Source: CAD feature listing. Evaluate the final solid. Frame: model axes, mm. A direction names the side the tool comes from. Coordinates: 2 decimals unless noted, no trailing zeros. Order: outer loops, then holes, each group sorted by start corner. A loop starts at its lowest first (then second) coordinate and runs counter-clockwise, first axis right, second up. Notation, with made-up numbers: (57, 47) -> (102, 47) arc R33 ccw to (102, 76) -> close; hole circle Ø6 at (-10, 80.5). An arc over 180 degrees is marked (long way). Put each result on its own line as item: value.
from build123d import *

# Parameters (mm, degrees)
SKETCH1_W                 = 465.838
SKETCH1_H                 = 365.232
BOSS_EXTRUDE1_DEPTH       = 3.175
SKETCH2_W                 = 465.838
SKETCH2_H                 = 365.232
SKETCH2_W_2               = 459.488
SKETCH2_H_2               = 47.625
SKETCH2_W_3               = 89.789
SKETCH2_H_3               = 308.082
SKETCH2_W_4               = 87.632
BOSS_EXTRUDE2_DEPTH       = 200.6
BOSS_EXTRUDE5_OUTLINE_W   = 87.632
BOSS_EXTRUDE5_OUTLINE_H   = 308.082
BOSS_EXTRUDE5_OUTLINE_W_2 = 89.789
BOSS_EXTRUDE5_DEPTH       = 38.1
CUT_EXTRUDE2_DEPTH        = 35
BOSS_EXTRUDE6_DEPTH       = 30.8
CUT_EXTRUDE3_DEPTH        = 579.469838561
SKETCH10_W                = 34.036
SKETCH10_H                = 101.6
SKETCH10_W_2              = 50.8
SKETCH10_H_2              = 34.036
BOSS_EXTRUDE7_DEPTH       = 3.175


# Read off the part's stored shape, not the designer's step: Boss-Extrude5
with BuildPart() as part:
    # Sketch1 → Boss-Extrude1 (new body)
    with BuildSketch(Plane.XY):
        with Locations((-46.4825, -25.4)):
            Rectangle(SKETCH1_W, SKETCH1_H)
    extrude(amount=BOSS_EXTRUDE1_DEPTH)

    # Sketch2 → Boss-Extrude2 (add)
    with BuildSketch(Plane.XY.offset(3.175)):
        with Locations((-46.4825, -25.4)):
            Rectangle(SKETCH2_W, SKETCH2_H)
        with Locations((-46.4825, -181.0285)):
            Rectangle(SKETCH2_W_2, SKETCH2_H_2, mode=Mode.SUBTRACT)
        with Locations((138.367, 0)):
            Rectangle(SKETCH2_W_3, SKETCH2_H_3, mode=Mode.SUBTRACT)
        with Locations((45.403, 0)):
            Rectangle(SKETCH2_W_3, SKETCH2_H_3, mode=Mode.SUBTRACT)
        with Locations((-47.561, 0)):
            Rectangle(SKETCH2_W_3, SKETCH2_H_3, mode=Mode.SUBTRACT)
        with Locations((-140.525, 0)):
            Rectangle(SKETCH2_W_3, SKETCH2_H_3, mode=Mode.SUBTRACT)
        with Locations((-232.4105, 0)):
            Rectangle(SKETCH2_W_4, SKETCH2_H_3, mode=Mode.SUBTRACT)
    extrude(amount=BOSS_EXTRUDE2_DEPTH)

    # Boss-Extrude5 outline → Boss-Extrude5 (add)
    with BuildSketch(Plane.XY.offset(203.775)):
        Polygon((183.2615, -208.016), (186.4365, -208.016), (186.4365, 157.216), (-279.4015, 157.216), (-279.4015, -208.016), (-276.2265, -208.016), (-276.2265, -157.216), (183.2615, -157.216), align=None)
        with Locations((-232.4105, 0)):
            Rectangle(BOSS_EXTRUDE5_OUTLINE_W, BOSS_EXTRUDE5_OUTLINE_H, mode=Mode.SUBTRACT)
        with Locations((-140.525, 0)):
            Rectangle(BOSS_EXTRUDE5_OUTLINE_W_2, BOSS_EXTRUDE5_OUTLINE_H, mode=Mode.SUBTRACT)
        with Locations((-47.561, 0)):
            Rectangle(BOSS_EXTRUDE5_OUTLINE_W_2, BOSS_EXTRUDE5_OUTLINE_H, mode=Mode.SUBTRACT)
        with Locations((45.403, 0)):
            Rectangle(BOSS_EXTRUDE5_OUTLINE_W_2, BOSS_EXTRUDE5_OUTLINE_H, mode=Mode.SUBTRACT)
        with Locations((138.367, 0)):
            Rectangle(BOSS_EXTRUDE5_OUTLINE_W_2, BOSS_EXTRUDE5_OUTLINE_H, mode=Mode.SUBTRACT)
    extrude(amount=BOSS_EXTRUDE5_DEPTH)

    # Sketch7 → Cut-Extrude2 (cut)
    with BuildSketch(Plane.XY.offset(241.875)):
        Polygon((-185.4195, -154.041), (-185.4195, 154.041), (-188.5945, 154.041), (-188.5945, -154.041), (-276.2265, -154.041), (-276.2265, -157.216), (183.2615, -157.216), (183.2615, -154.041), (93.4725, -154.041), (93.4725, 154.041), (90.2975, 154.041), (90.2975, -154.041), (0.5085, -154.041), (0.5085, 154.041), (-2.6665, 154.041), (-2.6665, -154.041), (-92.4555, -154.041), (-92.4555, 154.041), (-95.6305, 154.041), (-95.6305, -154.041), align=None)
    extrude(amount=-CUT_EXTRUDE2_DEPTH, mode=Mode.SUBTRACT)

    # Sketch8 → Boss-Extrude6 (add)
    with BuildSketch(Plane.XY.offset(241.875)):
        Polygon((183.2615, 154.041), (183.2615, -208.016), (186.4365, -208.016), (186.4365, 157.216), (-279.4015, 157.216), (-279.4015, -208.016), (-276.2265, -208.016), (-276.2265, 154.041), align=None)
    extrude(amount=BOSS_EXTRUDE6_DEPTH)

    # Sketch9 → Cut-Extrude3 (cut, through all)
    with BuildSketch(Plane(origin=(186.4365, 0, 0), x_dir=(0, 0, -1), z_dir=(1, 0, 0))):
        Polygon((-272.675, -208.016), (-215.525, -208.016), (-272.675, -131.816), align=None)
        Polygon((-272.675, 157.216), (-272.675, 81.016), (-215.525, 157.216), align=None)
    extrude(amount=-CUT_EXTRUDE3_DEPTH, mode=Mode.SUBTRACT)

    # Sketch10 → Boss-Extrude7 (add)
    with BuildSketch(Plane.XY):
        with Locations((203.4545, 106.416)):
            Rectangle(SKETCH10_W, SKETCH10_H)
        with Locations((203.4545, -106.416)):
            Rectangle(SKETCH10_W, SKETCH10_H)
        with Locations((161.0365, 174.234)):
            Rectangle(SKETCH10_W_2, SKETCH10_H_2)
    boss_extrude7 = extrude(amount=BOSS_EXTRUDE7_DEPTH)

    # Mirror1: Boss-Extrude7 across plane
    add(boss_extrude7.mirror(Plane.ZY.offset(46.4825)))


solid = part.part
1. Cut plane D-D on y = -79. Output: boundary loops of the cut face in (x, z) (1 decimal).
Numbers:
outline: (-313.4, 0) -> (220.5, 0) -> (220.5, 3.2) -> (186.4, 3.2) -> (186.4, 272.7) -> (183.3, 272.7) -> (183.3, 3.2) -> (93.5, 3.2) -> (93.5, 206.9) -> (90.3, 206.9) -> (90.3, 3.2) -> (0.5, 3.2) -> (0.5, 206.9) -> (-2.7, 206.9) -> (-2.7, 3.2) -> (-92.5, 3.2) -> (-92.5, 206.9) -> (-95.6, 206.9) -> (-95.6, 3.2) -> (-185.4, 3.2) -> (-185.4, 206.9) -> (-188.6, 206.9) -> (-188.6, 3.2) -> (-276.2, 3.2) -> (-276.2, 272.7) -> (-279.4, 272.7) -> (-279.4, 3.2) -> (-313.4, 3.2) -> close
2. Cut plane C-C on z = 246.5. Output: boundary loops of the cut face in (x, y), plus the area to 3 significant figures.
Numbers:
outline: (-279.4, -166.72) -> (-276.23, -166.72) -> (-276.23, 115.92) -> (-279.4, 115.92) -> close; (183.26, -166.72) -> (186.44, -166.72) -> (186.44, 115.92) -> (183.26, 115.92) -> close
area: 1,790 mm2
3. Set-up query: faces 1 (the flat face through (90.298, -2, 104)), 2 (the flat face through (203, 107, 3.175)), 3 (the flat face through (-296, -106, 3.175)). Return all of +Z, -Z, +X, -X, +Y, -Y with unobstructed straight access to the full face (end or side cutting, diameter ignored); none if empty.
Numbers:
face 1: +Z
face 2: +Z, +X, +Y, -Y
face 3: +Z, -X, +Y, -Y
4. Cut plane B-B on y = 40.5. Output: boundary loops of the cut face in (x, z) (1 decimal), plus the area to 3 significant figures.
Numbers:
outline: (-279.4, 0) -> (186.4, 0) -> (186.4, 272.7) -> (183.3, 272.7) -> (183.3, 3.2) -> (93.5, 3.2) -> (93.5, 206.9) -> (90.3, 206.9) -> (90.3, 3.2) -> (0.5, 3.2) -> (0.5, 206.9) -> (-2.7, 206.9) -> (-2.7, 3.2) -> (-92.5, 3.2) -> (-92.5, 206.9) -> (-95.6, 206.9) -> (-95.6, 3.2) -> (-185.4, 3.2) -> (-185.4, 206.9) -> (-188.6, 206.9) -> (-188.6, 3.2) -> (-276.2, 3.2) -> (-276.2, 272.7) -> (-279.4, 272.7) -> close
area: 5,780 mm2
5. Ray query, line 1 along Y through (x, z) = (177.5, 188); line 2 along X through (y, z) = (-33.5, 128); line 3 along X through (y, z) = (-176, 121). Return the intervals inside material, ascending.
Numbers:
line 1: y = -208.02 to -204.84, -157.22 to -154.04, 154.04 to 157.22
line 2: x = -279.4 to -276.23, -188.59 to -185.42, -95.63 to -92.46, -2.67 to 0.51, 90.3 to 93.47, 183.26 to 186.44
line 3: x = -279.4 to -276.23, 183.26 to 186.44
6. First-contact query: pin 1 (2.5 mm diameter, centred on x = -288.5, z = 2, fed in from -Y); pin 2 (2.5 mm diameter, centred on x = 204.5, z = 1.5, fed in from +Y); pin 3 (1 mm diameter, centred on y = 181, z = 1.5, fed in from -X). Flat tips, straight axial feed; report the tip coordinate or a pass-through.
Numbers:
pin 1: stops at y = -157.22
pin 2: stops at y = 157.22
pin 3: stops at x = -279.4
7. Pull-direction query (Y, two-part tool) for faces 4 (the flat face through (-45.396, 155.627, 216.717)), 5 (the flat face through (-188.594, -2, 104)), 6 (the flat face through (-43, -6, 0)), 7 (the flat face through (-277.79, -170.45, 243.7)); classes: pulls with the +Y half, pulls with the -Y half, needs draft (parallel to the pull), parting line crosses it, or undercut.
Numbers:
face 4: pulls with the +Y half
face 5: undercut
face 6: needs draft
face 7: pulls with the -Y half
8. Cut plane A-A on z = 167. Output: boundary loops of the cut face in (x, y), plus the area to 3 significant figures.
Numbers:
outline: (-279.4, -208.02) -> (186.44, -208.02) -> (186.44, 157.22) -> (-279.4, 157.22) -> close; hole (-276.23, -204.84) -> (183.26, -204.84) -> (183.26, -157.22) -> (-276.23, -157.22) -> close; hole (-276.23, -154.04) -> (-188.59, -154.04) -> (-188.59, 154.04) -> (-276.23, 154.04) -> close; hole (-185.42, -154.04) -> (-95.63, -154.04) -> (-95.63, 154.04) -> (-185.42, 154.04) -> close; hole (-92.46, -154.04) -> (-2.67, -154.04) -> (-2.67, 154.04) -> (-92.46, 154.04) -> close; hole (0.51, -154.04) -> (90.3, -154.04) -> (90.3, 154.04) -> (0.51, 154.04) -> close; hole (93.47, -154.04) -> (183.26, -154.04) -> (183.26, 154.04) -> (93.47, 154.04) -> close
area: 10,600 mm2
